CAD build for the part. Positions are in the model's coordinates, mm. A direction names the side the tool comes from. Give positions to 0.01 mm unless a question says otherwise; leave off trailing zeros. Write each loop counter-clockwise with the first axis right and the second up, starting at its lowest first coordinate (ties: lowest second). Pieces come first, ordered by that corner, then holes. Notation, with made-up numbers: (-19, 10.5) - (8, 10.5) arc R21 ccw to (8, 35.5) - close; hole circle Ø1 at (43.25, 10.25). An arc over 180 degrees is marked (long way). Answer as a JSON object with one key per item and string values.
from build123d import *

# Parameters (mm, degrees)
SKETCH_1_R          = 12.5
EXTRUDE_1_DEPTH     = 6
SKETCH_2_R          = 6
EXTRUDE_2_DEPTH     = 6
SKETCH_3_W          = 24
SKETCH_3_H          = 24
EXTRUDE_3_DEPTH     = 3
SKETCH_4_R          = 12.5
EXTRUDE_4_DEPTH     = 6
SKETCH_937_R        = 3
CUT_EXTRUDE_1_DEPTH = 28.449954463


with BuildPart() as part:
    # Эскиз1 → Бобышка-Вытянуть1 (new body)
    with BuildSketch(Plane.XY):
        Circle(SKETCH_1_R)
    extrude(amount=EXTRUDE_1_DEPTH)

    # Эскиз2 → Бобышка-Вытянуть2 (add)
    with BuildSketch(Plane(origin=(0, 0, 0), x_dir=(-1, 0, 0), z_dir=(0, 0, -1))):
        with Locations(Location((0, 0, 0), (0, 0, 180))):
            Circle(SKETCH_2_R)
    extrude(amount=EXTRUDE_2_DEPTH)

    # Эскиз3 → Бобышка-Вытянуть3 (add)
    with BuildSketch(Plane.XY.offset(6)):
        Rectangle(SKETCH_3_W, SKETCH_3_H)
    extrude(amount=EXTRUDE_3_DEPTH)

    # Эскиз4 → Бобышка-Вытянуть4 (add)
    with BuildSketch(Plane.XY.offset(9)):
        with Locations(Location((0, 0, 0), (0, 0, 196.260204708))):
            Circle(SKETCH_4_R)
    extrude(amount=EXTRUDE_4_DEPTH)

    # Sketch 937 → Вырез-Вытянуть1 (cut, through all)
    with BuildSketch(Plane(origin=(0, 0, -6), x_dir=(-1, 0, 0), z_dir=(0, 0, -1))):
        Circle(SKETCH_937_R)
    extrude(amount=-CUT_EXTRUDE_1_DEPTH, mode=Mode.SUBTRACT)


solid = part.part
(1) Probe L1, parallel to Z at x = -4.5, y = -5; L2, parallel to Y at x = 0, z = 1.75; L3, parallel to Z at x = 11, y = -9.5. List the from-to ranges inside material, lowest first. Write a range as [from, to].
Answer key:
{"L1": "z = [0, 15]", "L2": "y = [-12.5, -3], [3, 12.5]", "L3": "z = [6, 9]"}
(2) Saw through at C-C, the plane z = 9.5. Give the cut face in (x, y), and give its area (3 significant figures).
Answer key:
{"outline": "circle Ø25 at (0, 0); hole circle Ø6 at (0, 0)", "area": "463 mm²"}
(3) 3-axis set-ups, long thin cutter, end or side, ignore diameter. For faces 1 (the face through (10, -10, 6)), 2 (the face through (10, -10, 9)), 3 (the face through (10, 10, 6)), 4 (the face through (0, 12, 7)): which of +Z, -Z, +X, -X, +Y, -Y reach the whole face in a straight line?
Answer key:
{"face 1": "-Z, +X, -Y", "face 2": "+Z, +X, -Y", "face 3": "-Z, +X, +Y", "face 4": "+X, -X, +Y"}
(4) Flat gauge pins, fed straight in: P1, Ø1.5, axis at y = -7, z = 3, coming from the +X side; P2, Ø2.5, axis at x = -9.5, y = -7, coming from the -Z side; P3, Ø1, axis at y = -5, z = 8, coming from the +X side. Where does each tip first touch, or does it go through?
Answer key:
{"P1": "stops at x = 10.83", "P2": "stops at z = 0", "P3": "stops at x = 12"}
(5) Saw through at A-A, the plane y = 0. Give the cut face in (x, z).
Answer key:
{"outline": "(-12.5, 0) - (-6, 0) - (-6, -6) - (-3, -6) - (-3, 15) - (-12.5, 15) - (-12.5, 9) - (-12, 9) - (-12, 6) - (-12.5, 6) - close; (3, -6) - (6, -6) - (6, 0) - (12.5, 0) - (12.5, 6) - (12, 6) - (12, 9) - (12.5, 9) - (12.5, 15) - (3, 15) - close"}
(6) Saw through at D-D, the plane x = 5. Give the cut face in (y, z).
Answer key:
{"outline": "(-12, 6) - (-11.46, 6) - (-11.46, 0) - (-3.32, 0) - (-3.32, -6) - (3.32, -6) - (3.32, 0) - (11.46, 0) - (11.46, 6) - (12, 6) - (12, 9) - (11.46, 9) - (11.46, 15) - (-11.46, 15) - (-11.46, 9) - (-12, 9) - close"}
